Autodesk Inventor part; units mm, degrees
ref_plane "YZ Plane" through (0, 0, 0) normal (1, 0, 0) x (0, 1, 0)
ref_plane "XZ Plane" through (0, 0, 0) normal (0, 1, 0) x (-1, 0, 0)
ref_plane "XY Plane" through (0, 0, 0) normal (0, 0, 1) x (1, 0, 0)
sketch "Sketch1" plane through (0, 0, 0) normal (0, 1, 0) x (-1, 0, 0)
  circle A0 centre (0, 0) radius 14.75
  circle A1 centre (0, 0) radius 18
  dimension "d0" = 29.5
  dimension "d1" = 36
extrude "Extrusion1" add sketch "Sketch1" along normal blind 11
thread "Thread1"
sketch "Sketch2" plane through (0, 0, 0) normal (0, -1, 0) x (1, 0, 0)
  circle A0 centre (0, 0) radius 14.75
  line L0 (-18.761, 1.7111) -> (-16.7388, 1.7111)
  line L1 (-16.7388, 1.7111) -> (-16.7388, -1.7889)
  line L2 (-16.7388, -1.7889) -> (-18.761, -1.7889)
  line L3 (-18.761, -1.7889) -> (-18.761, 1.7111)
  line L4 (-18.2148, -4.8087) -> (-16.3145, -4.1171)
  line L5 (-16.3145, -4.1171) -> (-15.1175, -7.406)
  line L6 (-15.1175, -7.406) -> (-17.0177, -8.0976)
  line L7 (-17.0177, -8.0976) -> (-18.2148, -4.8087)
  line L8 (-15.4716, -10.7485) -> (-13.9225, -9.4487)
  line L9 (-13.9225, -9.4487) -> (-11.6728, -12.1298)
  line L10 (-11.6728, -12.1298) -> (-13.2219, -13.4297)
  line L11 (-13.2219, -13.4297) -> (-15.4716, -10.7485)
  line L12 (-10.8624, -15.3919) -> (-9.8512, -13.6406)
  line L13 (-9.8512, -13.6406) -> (-6.8202, -15.3906)
  line L14 (-6.8202, -15.3906) -> (-7.8313, -17.1419)
  line L15 (-7.8313, -17.1419) -> (-10.8624, -15.3919)
  line L16 (-4.9429, -18.1788) -> (-4.5918, -16.1873)
  line L17 (-4.5918, -16.1873) -> (-1.1449, -16.7951)
  line L18 (-1.1449, -16.7951) -> (-1.4961, -18.7866)
  line L19 (-1.4961, -18.7866) -> (-4.9429, -18.1788)
  line L20 (1.5727, -18.7731) -> (1.2215, -16.7816)
  line L21 (1.2215, -16.7816) -> (4.6684, -16.1738)
  line L22 (4.6684, -16.1738) -> (5.0195, -18.1653)
  line L23 (5.0195, -18.1653) -> (1.5727, -18.7731)
  line L24 (7.8986, -17.103) -> (6.8875, -15.3517)
  line L25 (6.8875, -15.3517) -> (9.9186, -13.6017)
  line L26 (9.9186, -13.6017) -> (10.9297, -15.353)
  line L27 (10.9297, -15.353) -> (7.8986, -17.103)
  line L28 (13.2719, -13.3701) -> (11.7228, -12.0703)
  line L29 (11.7228, -12.0703) -> (13.9725, -9.3891)
  line L30 (13.9725, -9.3891) -> (15.5216, -10.689)
  line L31 (15.5216, -10.689) -> (13.2719, -13.3701)
  line L32 (17.0443, -8.0246) -> (15.1441, -7.3329)
  line L33 (15.1441, -7.3329) -> (16.3411, -4.044)
  line L34 (16.3411, -4.044) -> (18.2414, -4.7356)
  line L35 (18.2414, -4.7356) -> (17.0443, -8.0246)
  line L36 (18.761, -1.7111) -> (16.7388, -1.7111)
  line L37 (16.7388, -1.7111) -> (16.7388, 1.7889)
  line L38 (16.7388, 1.7889) -> (18.761, 1.7889)
  line L39 (18.761, 1.7889) -> (18.761, -1.7111)
  line L40 (18.2148, 4.8087) -> (16.3145, 4.1171)
  line L41 (16.3145, 4.1171) -> (15.1175, 7.406)
  line L42 (15.1175, 7.406) -> (17.0177, 8.0976)
  line L43 (17.0177, 8.0976) -> (18.2148, 4.8087)
  line L44 (15.4716, 10.7485) -> (13.9225, 9.4487)
  line L45 (13.9225, 9.4487) -> (11.6728, 12.1298)
  line L46 (11.6728, 12.1298) -> (13.2219, 13.4297)
  line L47 (13.2219, 13.4297) -> (15.4716, 10.7485)
  line L48 (10.8624, 15.3919) -> (9.8512, 13.6406)
  line L49 (9.8512, 13.6406) -> (6.8202, 15.3906)
  line L50 (6.8202, 15.3906) -> (7.8313, 17.1419)
  line L51 (7.8313, 17.1419) -> (10.8624, 15.3919)
  line L52 (4.9429, 18.1788) -> (4.5918, 16.1873)
  line L53 (4.5918, 16.1873) -> (1.1449, 16.7951)
  line L54 (1.1449, 16.7951) -> (1.4961, 18.7866)
  line L55 (1.4961, 18.7866) -> (4.9429, 18.1788)
  line L56 (-1.5727, 18.7731) -> (-1.2215, 16.7816)
  line L57 (-1.2215, 16.7816) -> (-4.6684, 16.1738)
  line L58 (-4.6684, 16.1738) -> (-5.0195, 18.1653)
  line L59 (-5.0195, 18.1653) -> (-1.5727, 18.7731)
  line L60 (-7.8986, 17.103) -> (-6.8875, 15.3517)
  line L61 (-6.8875, 15.3517) -> (-9.9186, 13.6017)
  line L62 (-9.9186, 13.6017) -> (-10.9297, 15.353)
  line L63 (-10.9297, 15.353) -> (-7.8986, 17.103)
  line L64 (-13.2719, 13.3701) -> (-11.7228, 12.0703)
  line L65 (-11.7228, 12.0703) -> (-13.9725, 9.3891)
  line L66 (-13.9725, 9.3891) -> (-15.5216, 10.689)
  line L67 (-15.5216, 10.689) -> (-13.2719, 13.3701)
  line L68 (-17.0443, 8.0246) -> (-15.1441, 7.3329)
  line L69 (-15.1441, 7.3329) -> (-16.3411, 4.044)
  line L70 (-16.3411, 4.044) -> (-18.2414, 4.7356)
  line L71 (-18.2414, 4.7356) -> (-17.0443, 8.0246)
  dimension "d6" = 3.5
  dimension "d10" = 360
extrude "Extrusion2" cut sketch "Sketch2" against normal blind 8 contours L0 L1 L2 L3 | L4 L5 L6 L7 | L8 L9 L10 L11 | L12 L13 L14 L15 | L16 L17 L18 L19 | L20 L21 L22 L23 | L24 L25 L26 L27 | L28 L29 L30 L31 | L32 L33 L34 L35 | L36 L37 L38 L39 | L40 L41 L42 L43 | L44 L45 L46 L47 | L48 L49 L50 L51 | L52 L53 L54 L55 | L56 L57 L58 L59 | L60 L61 L62 L63 | L64 L65 L66 L67 | L68 L69 L70 L71
properties part number "OBSN-30-B_ring" material "Nylon 6"
Check sheet for the modelled part. Datum: model origin and axes. Units: mm. A direction names the side the tool comes from. Coordinates: 2 decimals unless noted, no trailing zeros. Loops run counter-clockwise (first coordinate to the right, second up) from the corner with the lowest first, then second, coordinate; pieces in that order, holes last. Notation, with made-up numbers: (-16, 70) -> (30, 70) arc R17 cw to (30, 75) -> close; hole circle Ø6 at (31.25, 13.5). An arc over 180 degrees is marked (long way). Write item = value, one per line. Start each with the question number.
1. Section check D-D on x = -9. Record the cut outline in (y, z).
2. Draft check along Z on faces 4 (the flat face through (10.208, 3.944, -14.102)), 5 (the flat face through (15, 11, 0)), 6 (the flat face through (-8.36, 3.94, -14.5)). Enter one of: released by +Z, released by -Z, zero draft, split by the parting line, or undercut.
3. Depth check by flat-ended pin: P1, Ø3, axis at x = -14.5, y = 4, coming from the +Z side; P2, Ø4, axis at x = -4.5, z = 12, coming from the -Y side; P3, Ø0.8, axis at x = -9.5, z = -15.5, coming from the -Y side; P4, Ø3, axis at y = 2.5, z = 0.5, coming from the -X side. Enter the tip coordinate at first touch or a pass-through.
4. Section check C-C on y = 9.75. Record the cut outline in (x, z), then the cut area to 3 significant figures.
5. Section check B-B on z = 0. Record the cut outline in (x, y).
6. Section check A-A on x = 0. Record the cut outline in (y, z), then the cut area to 3 significant figures.
7. Tool access check on faces 1 (the flat face through (-16.88, 3.94, 4.24)), 2 (the flat face through (8.38, 3.94, -14.49)), 3 (the flat face through (17, 4, 1.789)). Record the directions out of +Z, -Z, +X, -X, +Y, -Y that give a thin tool (end or side, any length) a straight path to the whole face; none if there is none.
8. Material ranges on line 1 (Z direction, x = -7, y = 4.5); line 2 (Z direction, x = 7, y = 7.5); line 3 (Z direction, x = 0, y = 6.75), recorded low to high.
Responses:
q1.outline = (0, -14.13) -> (8, -14.13) -> (8, -15.59) -> (11, -15.59) -> (11, -11.69) -> (0, -11.69) -> close; (0, 11.69) -> (11, 11.69) -> (11, 15.59) -> (8, 15.59) -> (8, 14.13) -> (0, 14.13) -> close
q2.face_4 = released by -Z
q2.face_5 = zero draft
q2.face_6 = undercut
q3.P1 = 10.55
q3.P2 = 0
q3.P3 = 8
q3.P4 = -17.92
q4.outline = circle Ø36 at (0, 0); hole circle Ø29.5 at (0, 0)
q4.area = 334 mm2
q5.outline = (-18, 8) -> (-16.74, 8) -> (-16.74, 0) -> (-14.75, 0) -> (-14.75, 11) -> (-18, 11) -> close; (14.75, 0) -> (16.74, 0) -> (16.74, 8) -> (18, 8) -> (18, 11) -> (14.75, 11) -> close
q6.outline = (0, -18) -> (11, -18) -> (11, -14.75) -> (0, -14.75) -> close; (0, 14.75) -> (11, 14.75) -> (11, 18) -> (0, 18) -> close
q6.area = 71.5 mm2
q7.face_1 = +Z, -Y
q7.face_2 = -Y
q7.face_3 = +X, -Y
q8.line_1 = -16.58 to -15.7, -15.29 to -12.98, 12.98 to 15.29, 15.55 to 16.58
q8.line_2 = -16.58 to -15.55, -15.29 to -12.98, 12.98 to 15.29, 15.7 to 16.58
q8.line_3 = -18 to -14.75, 14.75 to 18
